from build123d import *

# Parameters (mm, degrees)
PAD_DEPTH    = 1
PAD004_DEPTH = 20
FILLET_R     = 10
FILLET001_R  = 2
SKETCH003_R  = 2
POCKET_DEPTH = 49.6274


with BuildPart() as part:
    # Sketch → Pad (new body)
    with BuildSketch(Plane.XY):
        with BuildLine():
            ThreePointArc((0, 65), (-39.250322, 51.811314), (-62.572638, 17.5973))
            ThreePointArc((-62.572638, 17.5973), (-62.281657, 16.256919), (-61.1956, 15.4192))
            Line((-61.1956, 15.4192), (-48.0942, 15.4192))
            ThreePointArc((-48.0942, 15.4192), (-46.017568, 16.268418), (-44.521334, 17.9402))
            ThreePointArc((44.629065, 17.6705), (0.14521, 47.99978), (-44.521334, 17.9402))
            ThreePointArc((44.629065, 17.6705), (45.695788, 16.297968), (47.167959, 15.3736))
            Line((47.167959, 15.3736), (54.923211, 15.384158))
            ThreePointArc((54.923211, 15.384158), (76.110008, 24.185371), (84.88237, 45.38413))
            Line((84.88237, 59.61183), (84.88237, 45.38413))
            ThreePointArc((84.88237, 59.61183), (83.304212, 63.421842), (79.4942, 65))
            Line((0, 65), (79.4942, 65))
        make_face()
    extrude(amount=PAD_DEPTH)

    # Sketch001 → Pad004 (new body)
    with BuildSketch(Plane.XY.offset(1)):
        with BuildLine():
            ThreePointArc((6e-05, 65), (-39.693641, 51.472467), (-62.865542, 16.5204))
            Line((-62.865542, 16.5204), (-59.765542, 16.5204))
            ThreePointArc((6e-05, 63), (-37.80132, 49.942273), (-59.765542, 16.5204))
            Line((80.00006, 63), (6e-05, 63))
            Line((80.00006, 65), (80.00006, 63))
            Line((6e-05, 65), (80.00006, 65))
        make_face()
    extrude(amount=PAD004_DEPTH)

    # Fillet
    fillet_edges = [part.edges().sort_by_distance(p)[0] for p in [
        (80.00006, 64, 21),
    ]]
    fillet(fillet_edges, radius=FILLET_R)

    # Fillet001
    fillet001_edges = [part.edges().sort_by_distance(p)[0] for p in [
        (-61.315542, 16.5204, 21),
    ]]
    fillet(fillet001_edges, radius=FILLET001_R)

    # Sketch003 → Pocket (cut, through all)
    with BuildSketch(Plane(origin=(0, 65, 0), x_dir=(-1, 0, 0), z_dir=(0, 1, 0))):
        with Locations((-42.40006, 15.5)):
            Circle(SKETCH003_R)
        with Locations((-28.50006, 15.5)):
            Circle(SKETCH003_R)
        with Locations((-14.50006, 15.5)):
            Circle(SKETCH003_R)
    extrude(amount=-POCKET_DEPTH, mode=Mode.SUBTRACT)


solid = part.part
Work out the finished part from the listing and answer in its coordinate system (mm). A direction names the side the tool comes from. Round coordinates to 2 decimals unless told otherwise and drop trailing zeros. Order: outer loops, then holes, each group sorted by start corner. A loop starts at its lowest first (then second) coordinate and runs counter-clockwise, first axis right, second up. Notation, with made-up numbers: M -34,-6 L 25,-6 A9 cw 25,7 Z; hole C 60,-26.75 d7. An arc over 180 degrees is marked long. Put each result on its own line as item: value. Start each with the question number.
Q1. Section A-A, the plane z = 15.5 is taken. Write down the section's boundary in (x, y).
Q2. Section D-D, the plane x = -8 is taken. Write down the section's boundary in (y, z), and give its area (3 significant figures).
Q3. For a pull along X with two mould halves and no side action, classify faces 3 (the cylindrical face through (-46.044, 16.25, 0.493)), 4 (the flat face through (-61, 16.52, 10)), 5 (the cylindrical face through (14.76, 64.014, 17.483)), 6 (the cylindrical face through (-37.35, 50.29, 10.86)) as pulls with the +X half, pulls with the -X half, needs draft (parallel to the pull), parting line crosses it, or undercut.
Q4. Flat-ended cylindrical pins translate along their axes: pin 1 (6.5 mm diameter, centred on x = 42.4, z = 15.5, fed in from -Y); pin 2 (1.5 mm diameter, centred on y = 20.5, z = 14, fed in from +X); pin 3 (2.5 mm diameter, centred on x = -62, z = 9.5, fed in from -Y). Find the tip coordinate at first contact, or state that the pin passes through.
Q5. A tool of negligible diameter and unlimited length cuts with its end or side. For faces 1 (the cylindrical face through (75.876, 23.953, 0.493)), 2 (the flat face through (41, 63, 11)), from which of +Z, -Z, +X, -X, +Y, -Y can it reach the whole face along a straight path? Write none if from no direction.
Q6. Section B-B, the plane y = 23 is taken. Write down the section's boundary in (x, z).
Q7. Section C-C, the plane z = 6.75 is taken. Write down the section's boundary in (x, y), and give its area (3 significant figures).
Q8. Straight lines are drawn through the part: L1, parallel to Y at x = 75.5, z = 14; L2, parallel to Z at x = -2.5, y = 57; L3, parallel to X at y = 19, z = 13. For each, find the intervals that lie inside material, in ascending order. Write a range as [from, to].
Findings below:
1. outline: M -62.87,16.52 L -59.77,16.52 A62 cw 0,63 L 12.5,63 L 12.5,65 L 0,65 A65 ccw Z; M 16.5,63 L 26.5,63 L 26.5,65 L 16.5,65 Z; M 30.5,63 L 40.4,63 L 40.4,65 L 30.5,65 Z; M 44.4,63 L 78.93,63 L 78.93,65 L 44.4,65 Z
2. outline: M 47.33,0 L 64.51,0 L 64.51,21 L 62.45,21 L 62.45,1 L 47.33,1 Z
2. area: 58.3 mm^2
3. face 3: undercut
3. face 4: needs draft
3. face 5: undercut
3. face 6: pulls with the +X half
4. pin 1: stops at y = 63
4. pin 2: stops at x = -58.34
4. pin 3: stops at y = 16.52
5. face 1: +Z, -Z, +X, -Y
5. face 2: +Z, +X, -Y
6. outline: M -60.79,0 L -42.13,0 L -42.13,1 L -57.71,1 L -57.71,21 L -60.79,21 Z; M 42.13,0 L 74.86,0 L 74.86,1 L 42.13,1 Z
7. outline: M -62.87,16.52 L -59.77,16.52 A62 cw 0,63 L 80,63 L 80,65 L 0,65 A65 ccw Z
7. area: 361 mm^2
8. L1: y = [63, 65]
8. L2: z = [0, 1]
8. L3: x = [-62.16, -59.07]
